from build123d import *

# Parameters (mm, degrees)
SKETCH1_R           = 2
BOSS_EXTRUDE1_DEPTH = 10


with BuildPart() as part:
    # Sketch1 → Boss-Extrude1 (new body)
    with BuildSketch(Plane.XY):
        with BuildLine():
            Line((1.997609294, 14.746687389), (28.748065289, 28.326566036))
            ThreePointArc((28.748065289, 28.326566036), (30.805734405, 35.300748137), (23.724834089, 36.954250141))
            ThreePointArc((23.724834089, 36.954250141), (20.851278613, 36.124816425), (18.018383872, 37.083976864))
            add(Edge.make_bspline(
                [(27.096341183, 57.0558637), (-15.03027812, 61.190372697), (18.018383872, 37.083976864)],
                knots=[5.074507124, 5.074507124, 5.074507124, 7.365213451, 7.365213451, 7.365213451], degree=2, weights=[1, 0.41272448, 1]))
            Line((27.096341183, 57.0558637), (55.915354023, 54.227427195))
            ThreePointArc((55.915354023, 54.227427195), (58.317172637, 56.086683182), (56.599353473, 58.591610886))
            Line((56.599353473, 58.591610886), (28.633722858, 64.642950152))
            add(Edge.make_bspline(
                [(28.633722858, 64.642950152), (-24.600856245, 76.162107481), (-4.624928751, 25.368416784)],
                knots=[3.507798101, 3.507798101, 3.507798101, 5.909316529, 5.909316529, 5.909316529], degree=2, weights=[1, 0.361650033, 1]))
            ThreePointArc((-4.624928751, 25.368416784), (-4.281398653, 23.35476873), (-4.7718634, 21.371782158))
            ThreePointArc((-4.7718634, 21.371782158), (-3.762925605, 15.631661435), (1.997609294, 14.746687389))
        make_face()
        with Locations((-0.265703814, 19.205096721)):
            Circle(SKETCH1_R, mode=Mode.SUBTRACT)
        with Locations((26.484752181, 32.784975369)):
            Circle(SKETCH1_R, mode=Mode.SUBTRACT)
    extrude(amount=BOSS_EXTRUDE1_DEPTH)


solid = part.part
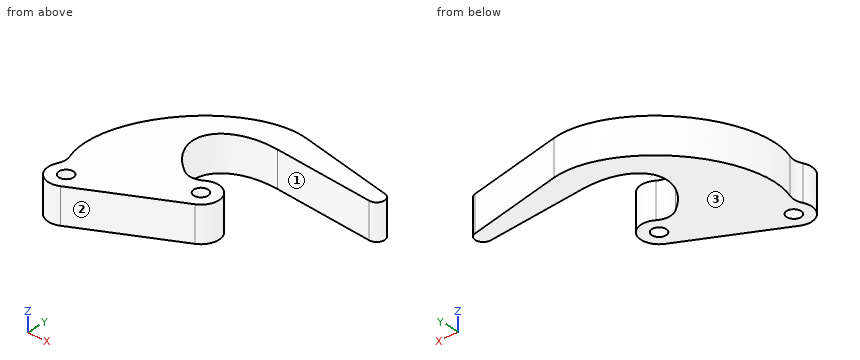
Input: part model. Units: mm. Frame: model coordinates. Face numbers are marked on the shaded views. Round coordinates to 2 decimals unless told otherwise and drop trailing zeros. Order: outer loops, then holes, each group sorted by start corner. A loop starts at its lowest first (then second) coordinate and runs counter-clockwise, first axis right, second up.
1. Cut plane A-A, the plane y = 23. Output: boundary loops of the cut face in (x, z).
The answers:
outline: (-4.31, 0) - (18.26, 0) - (18.26, 10) - (-4.31, 10) - close
2. Cut plane C-C, the plane z = 5.5. State how many separate pieces and enclosed holes the cut face has, then the cut area to 3 significant figures.
The answers:
separate pieces: 1
enclosed holes: 2
area: 1,170 mm2
3. Pin query (flat end, axial travel): P1, Ø1.5, axis at y = 47, z = 6.5, coming from the +X side; P2, Ø6, axis at y = 44, z = 7, coming from the -X side; P3, Ø1, axis at y = 49.5, z = 5.5, coming from the +X side (3 decimals). Return the tip coordinate at first contact, or that it passes through.
The answers:
P1: stops at x = 11.14
P2: stops at x = -4.6
P3: stops at x = 11.155
4. Material intervals for line 1 (Y direction, x = 13.5, z = 5.25); line 2 (Y direction, x = 15, z = 5.5); line 3 (X direction, y = 34.5, z = 7.25), sorted ascending.
The answers:
line 1: y = 20.59 to 41.42, 53.79 to 62.21
line 2: y = 21.35 to 39.69, 54.91 to 62.9
line 3: x = -5.88 to 25.46, 27.51 to 31.18
5. Cut plane B-B, the plane x = 37. Output: boundary loops of the cut face in (y, z).
The answers:
outline: (56.08, 0) - (62.83, 0) - (62.83, 10) - (56.08, 10) - close
6. Mould query, pull axis X, two halves, no side actions, for the marked faces 1, 2 and 3. Classes: released by +X, released by -X, zero draft, split by the parting line, or undercut.
The answers:
face 1: undercut
face 2: released by +X
face 3: zero draft
